Design review of the part built by this model. Coordinates are the model's own, in mm. Face numbers are marked on the shaded views. Give positions to 0.01 mm unless a question says otherwise; leave off trailing zeros. Loops run counter-clockwise (first coordinate to the right, second up) from the corner with the lowest first, then second, coordinate; pieces in that order, holes last. Notation, with made-up numbers: (-36, 89.5) - (22, 89.5) arc R13 ccw to (22, 97.5) - close; hole circle Ø7 at (23.5, 36.5). An arc over 180 degrees is marked (long way). Write each question's results on one line, items separated by ' | '.
```python
from build123d import *

# Parameters (mm, degrees)
SKETCH_2_R      = 10
SKETCH_3_R      = 22.5
EXTRUDE_1_DEPTH = 50


with BuildPart() as part:
    # По траектории1: sweep along a path in Эскиз1
    with BuildLine(Plane.XY) as sweep_1_path:
        Line((0, 0), (0, 200))
        ThreePointArc((0, 200), (65.444238832, 278.664666889), (154.703245421, 228.62560259))
        Line((154.703245421, 228.62560259), (161.859646068, 209.949791235))
    # Эскиз2 → По траектории1 (sweep)
    with BuildSketch(Plane(origin=(0, 0, 0), x_dir=(1, 0, 0), z_dir=(0, 1, 0))):
        Circle(SKETCH_2_R)
    sweep(path=sweep_1_path.line)

    # Эскиз3 → Бобышка-Вытянуть1 (add)
    with BuildSketch(Plane(origin=(0, 0, 0), x_dir=(1, 0, 0), z_dir=(0, 1, 0))):
        Circle(SKETCH_3_R)
    extrude(amount=EXTRUDE_1_DEPTH)


solid = part.part
```
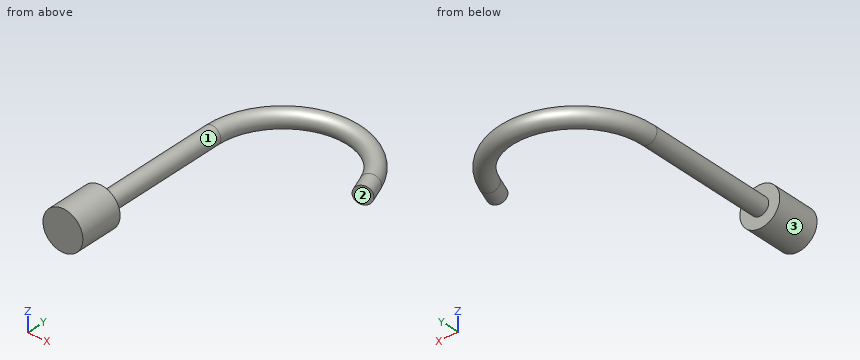
Item 1: Clearance check with flat-ended pins moving along their axes: P1, Ø10, axis at y = 223, z = 2.5, coming from the +X side; P2, Ø3, axis at x = 19.5, z = 12, coming from the +Y side; P3, Ø12, axis at x = 129.5, z = 8.5, coming from the +Y side. State where each tip first meets the part, or that it passes through.
Output values:
P1: stops at x = 169.34 | P2: stops at y = 50 | P3: stops at y = 276.69
Item 2: We need section D-D on z = 19. Give the boundary of the cut face in (x, y).
Output values:
outline: (-12.05, 0) - (12.05, 0) - (12.05, 50) - (-12.05, 50) - close
Item 3: Wall thickness on probe 1 along X at (y, z) = (45, -1.5); probe 2 along Y at (x, z) = (14.5, 17); probe 3 along X at (y, z) = (130, 0.5): over which ranges is each line inside the solid? List them lowest first.
Output values:
probe 1: x = -22.45 to 22.45 | probe 2: y = 0 to 50 | probe 3: x = -9.99 to 9.99
Item 4: Draft analysis for pull direction Y (two halves, no side actions). For the marked faces 1, 2 and 3, state which applies: +Y half, -Y half, draft (parallel to the pull), parting line (faces both ways), or undercut.
Output values:
face 1: undercut | face 2: -Y half | face 3: draft
Item 5: We need section B-B on y = 186. Give the boundary of the cut face in (x, z), then the cut area to 3 significant figures.
Output values:
outline: circle Ø20 at (0, 0) | area: 314 mm²
Item 6: We need section A-A on z = 0. Give the boundary of the cut face in (x, y).
Output values:
outline: (-22.5, 0) - (22.5, 0) - (22.5, 50) - (10, 50) - (10, 200) arc R70 cw to (145.37, 225.05) - (152.52, 206.37) - (171.2, 213.53) - (164.04, 232.2) arc R90 ccw to (-10, 200) - (-10, 50) - (-22.5, 50) - close
Item 7: We need section C-C on z = -18. Give the boundary of the cut face in (x, y).
Output values:
outline: (-13.5, 0) - (13.5, 0) - (13.5, 50) - (-13.5, 50) - close
